The model under review builds one solid part; all positions refer to its coordinate system, in mm. A direction names the side the tool comes from. Give positions to 0.01 mm unless a question says otherwise; leave off trailing zeros. Write item = value, one per line. Start each with the question number.
1. For faces 1 (the face through (-0.09, 2.152, -7.515)), 2 (the face through (-6.726, -4.984, -6.687)), 3 (the face through (8, -5, 0)), 4 (the face through (6.687, -4.984, -6.726)), list the 3-axis set-ups (+Z, -Z, +X, -X, +Y, -Y) from which the entire face can be reached by the end or side of a thin tool; tool diameter is ignored.
2. Wall thickness on line 1 along Z through (x, y) = (0, -3); line 2 along Y through (x, z) = (-2.5, -18.5); line 3 along Z through (x, y) = (0, -1.5): over which ranges is each line inside the solid? List them lowest first. Write a range as from..to.
3. For pin 1 (5 mm diameter, centred on y = -11.5, z = 6.5, fed in from -X); pin 2 (2 mm diameter, centred on y = -10, z = 0.5, fed in from +X); pin 3 (12 mm diameter, centred on x = -11, y = -10.5, fed in from +Z), all flat-tipped, find the tip position at first contact; note any pin that passes through.
4. Draft analysis for pull direction X (two halves, no side actions). For faces 5 (the face through (-0.34, 1.69, -2.62)), 6 (the face through (0, -5, 8)), 7 (the face through (-0.54, -1.95, 2.44)), 8 (the face through (-6.681, -4.975, 6.719)), state which applies: pulls with the +X half, pulls with the -X half, needs draft (parallel to the pull), parting line crosses it, or undercut.
from build123d import *

# Parameters (mm, degrees)
SKETCH4_W           = 17
SKETCH4_H           = 11
BOSS_EXTRUDE2_DEPTH = 8.5
CUT_EXTRUDE1_DEPTH  = 13.5
CUT_EXTRUDE2_DEPTH  = 13.5
CUT_EXTRUDE3_DEPTH  = 13.5
CUT_EXTRUDE4_DEPTH  = 13.5
FILLET1_R           = 2


with BuildPart() as part:
    # Sketch4 → Boss-Extrude2 (new body, symmetric)
    with BuildSketch(Plane.XY):
        Rectangle(SKETCH4_W, SKETCH4_H)
    extrude(amount=BOSS_EXTRUDE2_DEPTH, both=True)

    # Sketch5 → Cut-Extrude1 (cut, symmetric)
    with BuildSketch(Plane(origin=(0, 0, 0), x_dir=(0, 0, -1), z_dir=(1, 0, 0))):
        with BuildLine():
            Line((8.5, 5.5), (6.502509808, -1.291466653))
            ThreePointArc((6.502509808, -1.291466653), (6.473626767, -2.879228009), (7.259285969, -4.259285969))
            Line((7.259285969, -4.259285969), (8.5, -5.5))
            Line((8.5, -5.5), (8.5, 5.5))
        make_face()
        with BuildLine():
            Line((-8.5, -5.5), (-7.259285969, -4.259285969))
            ThreePointArc((-7.259285969, -4.259285969), (-6.473626767, -2.879228009), (-6.502509808, -1.291466653))
            Line((-6.502509808, -1.291466653), (-8.5, 5.5))
            Line((-8.5, 5.5), (-8.5, -5.5))
        make_face()
    extrude(amount=CUT_EXTRUDE1_DEPTH, both=True, mode=Mode.SUBTRACT)

    # Sketch7 → Cut-Extrude2 (cut, symmetric)
    with BuildSketch(Plane.XY):
        with BuildLine():
            Line((8.5, 5.5), (6.502538332, -1.291517059))
            ThreePointArc((6.502538332, -1.291517059), (6.473662442, -2.879270046), (7.259319467, -4.259319467))
            Line((7.259319467, -4.259319467), (8.5, -5.5))
            Line((8.5, -5.5), (8.5, 5.5))
        make_face()
        with BuildLine():
            Line((-8.5, -5.5), (-7.259319467, -4.259319467))
            ThreePointArc((-7.259319467, -4.259319467), (-6.473662442, -2.879270046), (-6.502538332, -1.291517059))
            Line((-6.502538332, -1.291517059), (-8.5, 5.5))
            Line((-8.5, 5.5), (-8.5, -5.5))
        make_face()
    extrude(amount=CUT_EXTRUDE2_DEPTH, both=True, mode=Mode.SUBTRACT)

    # Sketch11 → Cut-Extrude3 (cut, symmetric)
    with BuildSketch(Plane(origin=(0, 0, 0), x_dir=(0.707106781, 0, -0.707106781), z_dir=(0.707106781, 0, 0.707106781))):
        with BuildLine():
            Line((10, -5.5), (9.159523089, -4.659523089))
            ThreePointArc((9.159523089, -4.659523089), (8.341069319, -3.136306549), (8.499291869, -1.414382965))
            Line((8.499291869, -1.414382965), (9.693462893, 1.541294037))
            ThreePointArc((9.693462893, 1.541294037), (9.908907559, 2.799328578), (9.581873492, 4.033069244))
            ThreePointArc((9.581873492, 4.033069244), (9.013209006, 4.854851227), (8.25, 5.5))
            Line((8.25, 5.5), (14, 5.5))
            Line((14, 5.5), (14, -5.5))
            Line((14, -5.5), (10, -5.5))
        make_face()
        with BuildLine():
            Line((-14, 5.5), (-8.25, 5.5))
            ThreePointArc((-8.25, 5.5), (-9.013209006, 4.854851227), (-9.581873492, 4.033069244))
            ThreePointArc((-9.581873492, 4.033069244), (-9.908907559, 2.799328578), (-9.693462893, 1.541294037))
            Line((-9.693462893, 1.541294037), (-8.499291869, -1.414382965))
            ThreePointArc((-8.499291869, -1.414382965), (-8.341069319, -3.136306549), (-9.159523089, -4.659523089))
            Line((-9.159523089, -4.659523089), (-10, -5.5))
            Line((-10, -5.5), (-14, -5.5))
            Line((-14, -5.5), (-14, 5.5))
        make_face()
    extrude(amount=CUT_EXTRUDE3_DEPTH, both=True, mode=Mode.SUBTRACT)

    # Sketch12 → Cut-Extrude4 (cut, symmetric)
    with BuildSketch(Plane(origin=(0, 0, 0), x_dir=(-0.707106781, 0, -0.707106781), z_dir=(0.707106781, 0, -0.707106781))):
        with BuildLine():
            Line((10, -5.5), (9.159523089, -4.659523089))
            ThreePointArc((9.159523089, -4.659523089), (8.341069319, -3.136306549), (8.499291869, -1.414382965))
            Line((8.499291869, -1.414382965), (9.693462893, 1.541294037))
            ThreePointArc((9.693462893, 1.541294037), (9.908907559, 2.799328578), (9.581873492, 4.033069244))
            ThreePointArc((9.581873492, 4.033069244), (9.013209006, 4.854851227), (8.25, 5.5))
            Line((8.25, 5.5), (14, 5.5))
            Line((14, 5.5), (14, -5.5))
            Line((14, -5.5), (10, -5.5))
        make_face()
        with BuildLine():
            Line((-14, 5.5), (-8.25, 5.5))
            ThreePointArc((-8.25, 5.5), (-9.013209006, 4.854851227), (-9.581873492, 4.033069244))
            ThreePointArc((-9.581873492, 4.033069244), (-9.908907559, 2.799328578), (-9.693462893, 1.541294037))
            Line((-9.693462893, 1.541294037), (-8.499291869, -1.414382965))
            ThreePointArc((-8.499291869, -1.414382965), (-8.341069319, -3.136306549), (-9.159523089, -4.659523089))
            Line((-9.159523089, -4.659523089), (-10, -5.5))
            Line((-10, -5.5), (-14, -5.5))
            Line((-14, -5.5), (-14, 5.5))
        make_face()
    extrude(amount=CUT_EXTRUDE4_DEPTH, both=True, mode=Mode.SUBTRACT)

    # Sketch14 → Cut-Revolve1 (revolve, cut)
    with BuildSketch(Plane.XY):
        Polygon((0, 5.5), (5.5, 5.5), (2.5, 1.5), (2.5, -5.5), (0, -5.5), align=None)
    revolve(axis=Axis((0, -5.5, 0), (0, 1, 0)), mode=Mode.SUBTRACT)

    # Fillet1
    fillet1_edges = [part.edges().sort_by_distance(p)[0] for p in [
        (5.833630945, 5.5, -5.833630945),
        (-5.833630945, 5.5, -5.833630945),
        (-5.833630945, 5.5, 5.833630945),
        (5.833630945, 5.5, 5.833630945),
    ]]
    fillet(fillet1_edges, radius=FILLET1_R)

    # Sketch15 → Revolve1 (revolve)
    with BuildSketch(Plane(origin=(0, 0, 0), x_dir=(0, 0, -1), z_dir=(1, 0, 0))):
        with BuildLine():
            Line((0, -15.5), (22.5, -15.5))
            ThreePointArc((22.5, -15.5), (17.455904629, -8.920713416), (9.9979998, -5.3))
            Line((9.9979998, -5.3), (0, -5.3))
            Line((0, -5.3), (0, -5.5))
            Line((0, -5.5), (0, -15.5))
        make_face()
    revolve(axis=Axis((0, -5.5, 0), (0, -1, 0)))


solid = part.part
Final values:
q1.face_1 = -Z, +X, -X
q1.face_2 = -Z, -X
q1.face_3 = +Z, -Z, +X
q1.face_4 = -Z, +X
q2.line_1 = -6.51..-2.5, 2.5..6.51
q2.line_2 = -15.5..-10
q2.line_3 = -6.45..-2.5, 2.5..6.45
q3.pin_1 = -20.91
q3.pin_2 = 19.6
q3.pin_3 = 21.15
q4.face_5 = undercut
q4.face_6 = needs draft
q4.face_7 = undercut
q4.face_8 = pulls with the -X half
